Here's the drawing with two shaded views (mm, measured from the low corner). I have some questions. A direction names the side the tool comes from. Coordinates: 2 decimals unless noted, no trailing zeros. Loops run counter-clockwise (first coordinate to the right, second up) from the corner with the lowest first, then second, coordinate; pieces in that order, holes last. Notation, with made-up numbers: (76.25, -40) -> (98.25, -40) arc R16 cw to (98.25, -31) -> close; hole circle Ø5 at (-29, 37.5). An arc over 180 degrees is marked (long way). Answer as a JSON object with one key per item and string values. Group by question number.
1) I want a section at D-D (x = 198). Write out the boundary of the cut face in (y, z).
2) I want a section at C-C (y = 50). Write out the boundary of the cut face in (x, z), then the cut area to 3 significant figures.
3) I'm going to push flat-ended pins straight in: pin 1 (5 mm diameter, centred on x = 150.5, y = 40, fed in from +Z); pin 2 (6 mm diameter, centred on x = 52, z = 56.5, fed in from +Y). Where does each tip first touch, or does it pass through?
4) I want a section at B-B (z = 173). Write out the boundary of the cut face in (x, y), then the cut area to 3 significant figures.
5) I want a section at A-A (x = 20). Write out the boundary of the cut face in (y, z).
6) Which directions (+Z, -Z, +X, -X, +Y, -Y) give clear straight access to the entire face, cutting with the end or side of a thin tool? Please do the marked faces 1 and 2.
7) I need wall thicknesses on probe 1 along Y at (x, z) = (20, 1); probe 2 along Z at (x, y) = (66.5, 62). Which ranges of each line are inside material? Lowest first, please. Write a range as [from, to].
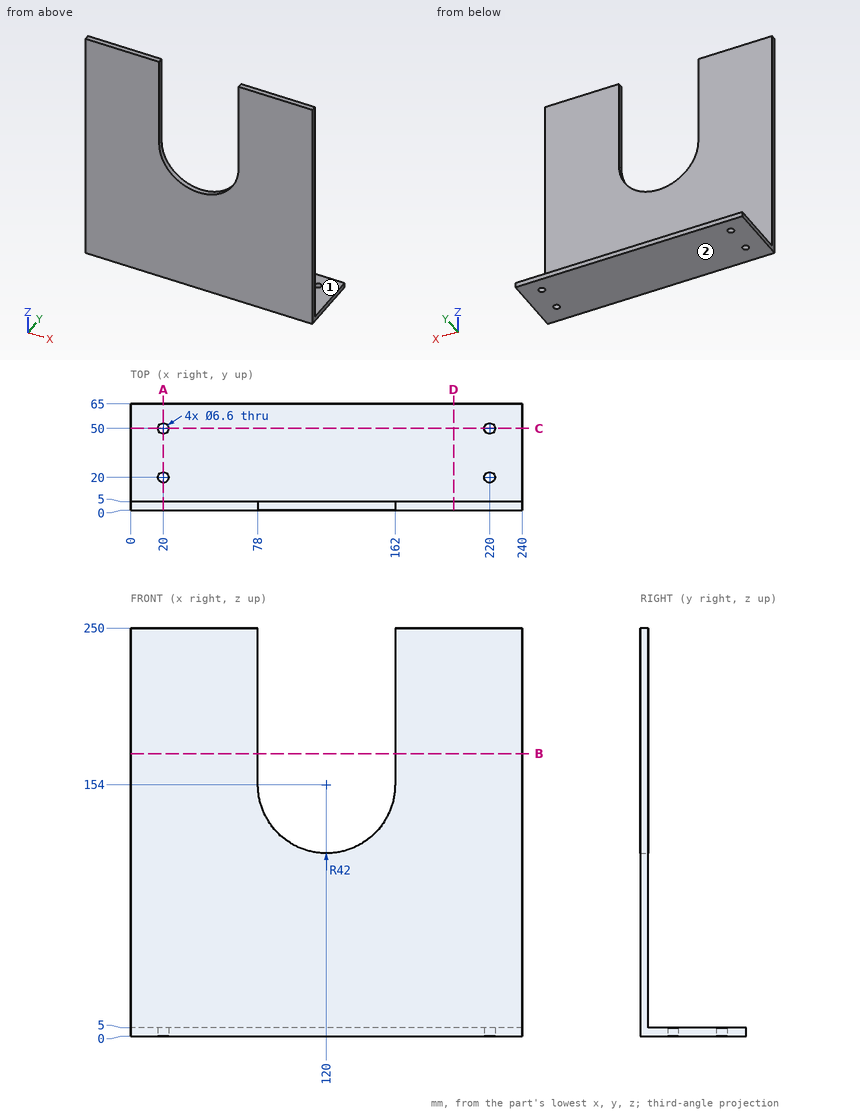
Determined:
{
 "1": {"outline": "(0, 0) -> (65, 0) -> (65, 5) -> (5, 5) -> (5, 250) -> (0, 250) -> close"},
 "2": {"outline": "(0, 0) -> (16.7, 0) -> (16.7, 5) -> (0, 5) -> close; (23.3, 0) -> (216.7, 0) -> (216.7, 5) -> (23.3, 5) -> close; (223.3, 0) -> (240, 0) -> (240, 5) -> (223.3, 5) -> close", "area": "1,130 mm^2"},
 "3": {"pin 1": "z = 5", "pin 2": "y = 5"},
 "4": {"outline": "(0, 0) -> (78, 0) -> (78, 5) -> (0, 5) -> close; (162, 0) -> (240, 0) -> (240, 5) -> (162, 5) -> close", "area": "780 mm^2"},
 "5": {"outline": "(0, 0) -> (16.7, 0) -> (16.7, 5) -> (5, 5) -> (5, 250) -> (0, 250) -> close; (23.3, 0) -> (46.7, 0) -> (46.7, 5) -> (23.3, 5) -> close; (53.3, 0) -> (65, 0) -> (65, 5) -> (53.3, 5) -> close"},
 "6": {"face 1": "+Z, +X, -X, +Y", "face 2": "-Z, +X, -X, +Y, -Y"},
 "7": {"probe 1": "[0, 16.7], [23.3, 46.7], [53.3, 65]", "probe 2": "[0, 5]"}
}
